Verification items for the finished model (mm, model axes). A direction names the side the tool comes from. Coordinates: 2 decimals unless noted, no trailing zeros. Loops run counter-clockwise (first coordinate to the right, second up) from the corner with the lowest first, then second, coordinate; pieces in that order, holes last. Notation, with made-up numbers: (89.25, 35) - (133.25, 35) arc R5 cw to (133.25, 42) - close; hole circle Ø11 at (-13.75, 67.5). An arc over 180 degrees is marked (long way). Answer as CSV lines item,"result". Start each with the question number.
1. Set-up check for faces 1 (the flat face through (-96, -11.988, 10)), 2 (the flat face through (-38.282, -21, 10)), 3 (the cylindrical face through (-93.874, -10.755, 4.601)): record each of +Z, -Z, +X, -X, +Y, -Y from which the full face is reachable in a straight line by a thin tool's end or side.
2. Cross-section at C-C (z = 13.25). Enter the section's corners in (x, y).
3. Cross-section at B-B (z = 4). Enter the section's corners in (x, y), plus the area to 3 significant figures.
4. Cross-section at D-D (x = -57). Enter the section's corners in (y, z).
5. Cross-section at A-A (y = -17.5). Enter the section's corners in (x, z).
6. Gauge pin test, flat ends, axial feed: P1, Ø5, axis at x = -95.782, z = 4, coming from the -Y side; P2, Ø1.5, axis at y = -25.5, z = 12, coming from the -X side; P3, Ø6, axis at x = -60, z = 9.5, coming from the +Y side. Record the tip position at first contact, or that the pin passes through.
7. Material ranges on line 1 (X direction, y = -16.25, z = 8.5); line 2 (Z direction, x = -96, y = -11); line 3 (X direction, y = -14.5, z = 19.25), recorded low to high. Write a range as [from, to].
8. Release check for a two-part mould opening along X. For faces 4 (the flat face through (-63, -27.315, 10)), 5 (the flat face through (-37, -14.815, 10)), 6 (the flat face through (-90.782, -21, 10)), 7 (the flat face through (-35.782, -22, 10)) record: pulls with the +X half, pulls with the -X half, needs draft (parallel to the pull), parting line crosses it, or undercut.
Autodesk Inventor part; units mm, degrees
ref_plane "YZ Plane" through (0, 0, 0) normal (1, 0, 0) x (0, 1, 0)
ref_plane "XZ Plane" through (0, 0, 0) normal (0, 1, 0) x (-1, 0, 0)
ref_plane "XY Plane" through (0, 0, 0) normal (0, 0, 1) x (1, 0, 0)
sketch "Sketch1" plane through (0, 0, 0) normal (0, 0, 1) x (1, 0, 0)
  line L0 (-100.782, -11.9876) -> (-90.782, -11.9876)
  line L1 (-100.782, -9.4876) -> (-88.282, -9.4876)
  line L2 (-90.782, -11.9876) -> (-90.782, -20.4134)
  line L3 (-88.282, -9.4876) -> (-88.282, -20.4134)
  line L4 (-90.782, -20.4134) -> (-90.782, -29.8154)
  line L5 (-90.782, -29.8154) -> (-35.782, -29.8154)
  line L6 (-35.782, -29.8154) -> (-35.782, -14.8154)
  line L7 (-38.282, -14.8154) -> (-38.282, -27.3154)
  line L8 (-38.282, -27.3154) -> (-88.282, -27.3154)
  line L9 (-88.282, -27.3154) -> (-88.282, -20.4134)
  line L10 (-100.782, -11.9876) -> (-100.782, -9.4876)
  line L11 (-35.782, -14.8154) -> (-38.282, -14.8154)
  dimension "d6" = 10
  dimension "d7" = 2.5
  dimension "d8" = 2.5
  dimension "d9" = 2.5
  dimension "d20" = 15
  dimension "d21" = 65
  dimension "d29" = 2.5
extrude "Extrusion1" add sketch "Sketch1" along normal blind 20
sketch "Sketch2" plane through (-100.782, -11.9876, 0) normal (0, -1, 0) x (1, 0, 0)
  line L0 (0, 0) -> (0, 20)
  line L1 (10, 0) -> (10, 20)
  line L2 (0, 20) -> (10, 20)
  line L3 (0, 0) -> (10, 0)
  circle A0 centre (5, 4) radius 2
  circle A1 centre (5, 16) radius 2
  line L4 (65, 0) -> (65, 20)
  point P0 (100.782, 0)
  dimension "d17" = 4
  dimension "d22" = 4
  dimension "d24" = 12
  dimension "d25" = 4
  dimension "d27" = 60
  dimension "d28" = 60
extrude "Extrusion2" cut sketch "Sketch2" against normal blind 4 contours A0 | A1
equation "\"d17\" = d22"
properties part number "Carcasa para Placa Reed Switch 40x20" material "ABS Plastic"
Values follow:
1,face 1,"+Z, -Z, -X, -Y"
1,face 2,"+Z, -Z, +Y"
1,face 3,"+Y, -Y"
2,outline,"(-100.78, -11.99) - (-90.78, -11.99) - (-90.78, -29.82) - (-35.78, -29.82) - (-35.78, -14.82) - (-38.28, -14.82) - (-38.28, -27.32) - (-88.28, -27.32) - (-88.28, -9.49) - (-100.78, -9.49) - close"
3,outline,"(-100.78, -11.99) - (-97.78, -11.99) - (-97.78, -9.49) - (-100.78, -9.49) - close; (-93.78, -11.99) - (-90.78, -11.99) - (-90.78, -29.82) - (-35.78, -29.82) - (-35.78, -14.82) - (-38.28, -14.82) - (-38.28, -27.32) - (-88.28, -27.32) - (-88.28, -9.49) - (-93.78, -9.49) - close"
3,area,"228 mm²"
4,outline,"(-29.82, 0) - (-27.32, 0) - (-27.32, 20) - (-29.82, 20) - close"
5,outline,"(-90.78, 0) - (-88.28, 0) - (-88.28, 20) - (-90.78, 20) - close; (-38.28, 0) - (-35.78, 0) - (-35.78, 20) - (-38.28, 20) - close"
6,P1,"stops at y = -11.99"
6,P2,"stops at x = -90.78"
6,P3,"stops at y = -27.32"
7,line 1,"x = [-90.78, -88.28], [-38.28, -35.78]"
7,line 2,"z = [0, 2.01], [5.99, 14.01], [17.99, 20]"
7,line 3,"x = [-90.78, -88.28]"
8,face 4,"undercut"
8,face 5,"needs draft"
8,face 6,"pulls with the -X half"
8,face 7,"pulls with the +X half"
